Could you check a few things on this model? Use its own coordinates, in mm. A direction names the side the tool comes from. Round coordinates to 2 decimals unless told otherwise and drop trailing zeros. Loops run counter-clockwise (first coordinate to the right, second up) from the corner with the lowest first, then second, coordinate; pieces in that order, holes last. Notation, with made-up numbers: (4, 34) -> (62, 34) arc R14 cw to (62, 59) -> close; hole circle Ø11 at (-36, -23). An arc over 180 degrees is marked (long way). One line per item, written item: value.
```python
from build123d import *

# Parameters (mm, degrees)
SKETCH3_R   = 21.828125
SKETCH3_R_2 = 13.3223


with BuildPart() as part:
    # Sketch1 → Revolve1 (revolve)
    with BuildSketch(Plane.XY):
        Polygon((6.801339045, -40.61975447), (17.432763151, -14.953226207), (12.636789012, -12.966668675), (2.181363958, -38.706098131), align=None)
    revolve(axis=Axis((-13.365218875, -32.266492673, 0), (0.382683432, 0.923879533, 0)))



with BuildPart() as body_2:
    # Sketch2 → Revolve2 (revolve)
    with BuildSketch(Plane.XY):
        Polygon((16.8275, 34.925), (16.637, 7.14375), (21.828125, 7.14375), (21.828125, 34.925), align=None)
    revolve(axis=Axis((0, 0, 0), (0, 1, 0)))


with BuildPart() as part_1:
    add(part.part)

    add(body_2.part)  # Sweep1 merges body 2
    # Sweep1: sweep along a path in Sketch4
    with BuildLine(Plane.XY) as sweep1_path:
        ThreePointArc((-2.73379477, -6.59996441), (-0.690078525, 0.137265153), (0, 7.14375))
    # Sketch3 → Sweep1 (sweep)
    with BuildSketch(Plane(origin=(-2.73379477, -6.59996441, 0), x_dir=(0, 0, -1), z_dir=(0.382683432, 0.923879533, 0))):
        Circle(SKETCH3_R)
        Circle(SKETCH3_R_2, mode=Mode.SUBTRACT)
    sweep(path=sweep1_path.line)


solid = part_1.part
```
(1) Imagine slicing it at A-A on y = 26.5. Write out the boundary of the cut face in (x, z), then the cut area to 3 significant figures.
Results below:
outline: circle Ø43.66 at (0, 0); hole circle Ø33.54 at (0, 0)
area: 613 mm²
(2) For pin 1 Ø3 at (x, y) = (-16, 20.5) entering from +Z; pin 2 Ø8 at (y, z) = (-5, 17) entering from +X; pin 3 Ø3 at (x, y) = (-24, 8.5) entering from -Z; pin 4 Ø8 at (x, z) = (15.5, -0.5) entering from +Y (3 decimals), each with a flat end and sliding along its axis, tell me the tip position at first contact or that it passes through.
Results below:
pin 1: stops at z = 16.32
pin 2: stops at x = 16.26
pin 3: passes through
pin 4: stops at y = 34.925
(3) Please list where these lines run through material, in increasing order: L1, parallel to X at y = -3.5, z = 11.5; L2, parallel to X at y = -25, z = -13; L3, parallel to Z at x = 0.5, y = 32.
Results below:
L1: x = -21.53 to -14.48, -10.22 to -8.74, 5.38 to 17.5
L2: x = -29.33 to -21.88, 1.07 to 8.62
L3: z = -21.82 to -16.8, 16.8 to 21.82
(4) We'd pull the mould along X, two halves only. Please class faces 4 (the face through (6.157, -25.528, 6.409)), 5 (the face through (-23.728, -27.974, 12.833)), 6 (the face through (-4.73, 21.23, 21.31)): +X half, -X half, draft (parallel to the pull), parting line (faces both ways), or undercut.
Results below:
face 4: undercut
face 5: -X half
face 6: parting line
(5) On a 3-axis mill with a long thin cutter (end or side, diameter ignored), from which of +Z, -Z, +X, -X, +Y, -Y can I reach the whole of each face in a straight line? I mean faces 1 (the face through (11, 34.925, 13)), 2 (the face through (-2.81, -6.57, -13.63)), 3 (the face through (-3.627, 20.84, 16.333)). Say none if no direction works.
Results below:
face 1: +Z, -Z, +X, -X, +Y
face 2: none
face 3: +Y
